from build123d import *

# Parameters (mm, degrees)
SKETCH_1_R               = 3.9
SKETCH_1_R_2             = 2.65
EXTRUDE_1_DEPTH          = 11
EXTRUDE_START            = -3
SKETCH_2_R               = 2.65
EXTRUDE_2_DEPTH          = 3
EXTRUDE_START_2          = 6.2
EXTRUDE_3_DEPTH          = 6.2
CHAMFER_1_SIZE           = 0.3
CHAMFER_2_SIZE           = 0.3
EXTRUDE_4_DEPTH          = 1
EXTRUDE_4_DEPTH_BACK     = 2
SKETCH_4_R               = 13.9
SKETCH_5_R               = 4.9
SKETCH_5_R_2             = 3.7
EXTRUDE_5_DEPTH          = 5
CHAMFER_4_SIZE           = 2
CUT_EXTRUDE_1_DEPTH      = 22.619898242
CUT_EXTRUDE_1_DEPTH_BACK = 22.619898242
SKETCH_6_R               = 1.5
CHAMFER_5_SIZE           = 1
CHAMFER_6_SIZE           = 1


with BuildPart() as part:
    # 草图1 → 凸台-拉伸1 (new body)
    with BuildSketch(Plane.XY):
        Circle(SKETCH_1_R)
        Circle(SKETCH_1_R_2, mode=Mode.SUBTRACT)
    extrude(amount=EXTRUDE_1_DEPTH)

    # 草图2 → 凸台-拉伸2 (add)
    with BuildSketch(Plane.XY.offset(11).offset(EXTRUDE_START)):
        Circle(SKETCH_2_R)
    extrude(amount=EXTRUDE_2_DEPTH)

    # 草图3 → 凸台-拉伸3 (add)
    with BuildSketch(Plane(origin=(0, 0, 8), x_dir=(-1, 0, 0), z_dir=(0, 0, -1)).offset(EXTRUDE_START_2)):
        with BuildLine():
            Line((-1.65, -2.073644135), (-1.65, 2.073644135))
            ThreePointArc((-1.65, 2.073644135), (-2.65, 0), (-1.65, -2.073644135))
        make_face()
        with BuildLine():
            ThreePointArc((2.65, 0), (2.386943652, 1.151086443), (1.65, 2.073644135))
            Line((1.65, 2.073644135), (1.65, -2.073644135))
            ThreePointArc((1.65, -2.073644135), (2.386943652, -1.151086443), (2.65, 0))
        make_face()
    extrude(amount=-EXTRUDE_3_DEPTH)

    # 倒角1
    chamfer_1_edges = [part.edges().sort_by_distance(p)[0] for p in [
        (-2.65, 0, 0),
    ]]
    chamfer(chamfer_1_edges, length=CHAMFER_1_SIZE)

    # 倒角2
    chamfer_2_edges = [part.edges().sort_by_distance(p)[0] for p in [
        (-3.9, 0, 0),
    ]]
    chamfer(chamfer_2_edges, length=CHAMFER_2_SIZE)

    # 草图4 → 凸台-拉伸4 (add, two sides: drawn at the far end of the back side and taken through both)
    with BuildSketch(Plane.XY.offset(11).offset(-EXTRUDE_4_DEPTH_BACK)):
        Circle(SKETCH_4_R)
    extrude(amount=EXTRUDE_4_DEPTH + EXTRUDE_4_DEPTH_BACK)

    # 草图5 → 凸台-拉伸5 (add)
    with BuildSketch(Plane(origin=(0, 0, 9), x_dir=(-1, 0, 0), z_dir=(0, 0, -1))):
        with Locations(Location((0, 0, 0), (0, 0, 180))):
            Circle(SKETCH_5_R)
        Circle(SKETCH_5_R_2, mode=Mode.SUBTRACT)
    extrude(amount=EXTRUDE_5_DEPTH)

    # 倒角4
    chamfer_4_edges = [part.edges().sort_by_distance(p)[0] for p in [
        (-13.9, 0, 9),
    ]]
    chamfer(chamfer_4_edges, length=CHAMFER_4_SIZE)

    # 草图6 → 切除-拉伸1 (cut, two sides: drawn at the far end of the back side and taken through both)
    with BuildSketch(Plane(origin=(0, 0, 9), x_dir=(-1, 0, 0), z_dir=(0, 0, -1)).offset(-CUT_EXTRUDE_1_DEPTH_BACK)):
        with Locations((0, 6)):
            Circle(SKETCH_6_R)
        with Locations((5.196152423, 3)):
            Circle(SKETCH_6_R)
        with Locations((5.196152423, -3)):
            Circle(SKETCH_6_R)
        with Locations((0, -6)):
            Circle(SKETCH_6_R)
        with Locations((-5.196152423, -3)):
            Circle(SKETCH_6_R)
        with Locations((-5.196152423, 3)):
            Circle(SKETCH_6_R)
    extrude(amount=CUT_EXTRUDE_1_DEPTH + CUT_EXTRUDE_1_DEPTH_BACK, mode=Mode.SUBTRACT)

    # 倒角5
    chamfer_5_edges = [part.edges().sort_by_distance(p)[0] for p in [
        (-1.65, 0, 1.8),
    ]]
    chamfer(chamfer_5_edges, length=CHAMFER_5_SIZE - 0.0001)  # a hair under: the kernel refuses the full size

    # 倒角6
    chamfer_6_edges = [part.edges().sort_by_distance(p)[0] for p in [
        (1.65, 0, 1.8),
    ]]
    chamfer(chamfer_6_edges, length=CHAMFER_6_SIZE - 0.0001)  # a hair under: the kernel refuses the full size


solid = part.part
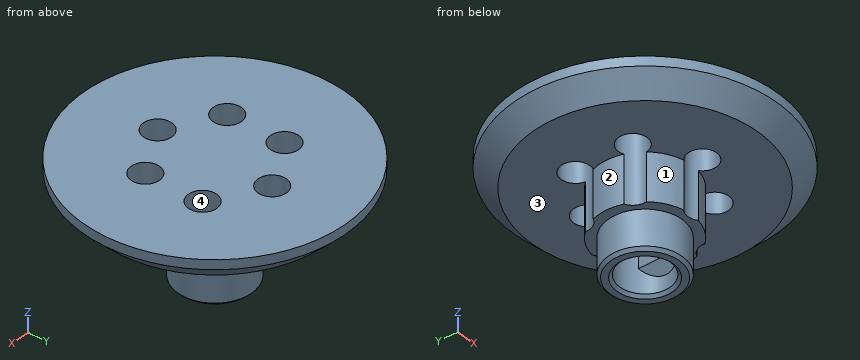
The listing builds one solid part. Answer for the finished solid, in the listing's coordinates (mm). Face numbers are marked on the shaded views. A direction names the side the tool comes from. Coordinates: 2 decimals unless noted, no trailing zeros. Order: outer loops, then holes, each group sorted by start corner. A loop starts at its lowest first (then second) coordinate and runs counter-clockwise, first axis right, second up.
Q1. Consider line 1 (Y direction, x = 0, z = 5.75); line 2 (X direction, y = 3, z = 10.25); line 3 (Y direction, x = -4.25, z = 9.75). Determine where each line is inside the solid, lowest interval first.
Q2. A cutting plane is placed at B-B, the plane z = 7. Write down the section's boundary in (x, y).
Q3. Which of the six approach directions +Z, -Z, +X, -X, +Y, -Y give full straight-line access (tool end or side, diameter ignored) to the marked faces 1, 2, 3 and 4?
Q4. A cutting plane is placed at A-A, the plane z = 9.5. Write down the section's boundary in (x, y), and give its area (3 significant figures).
Q5. Given P1, Ø4, axis at x = 5.2, y = -3, coming from the -Z side; P2, Ø1.5, axis at x = 3, z = 1.5, coming from the +Y side; P3, Ø6, axis at y = -6, z = 9, coming from the +X side; P4, Ø2.5, axis at x = 0, y = -6, coming from the +Z side, each flat-ended and moving along its own axis, determine where each tip first touches the part or whether it passes through.
Answers follow:
1. line 1: y = -4.5 to -2.65, 2.65 to 4.5
1. line 2: x = -12.8 to -6.7, -3.7 to 3.7, 6.7 to 12.8
1. line 3: y = -11.91 to -4.16, -1.84 to 1.84, 4.16 to 11.91
2. outline: (-4.63, -1.61) arc R1.5 cw to (-3.71, -3.2) arc R4.9 ccw to (-0.92, -4.81) arc R1.5 cw to (0.92, -4.81) arc R4.9 ccw to (3.71, -3.2) arc R1.5 cw to (4.63, -1.61) arc R4.9 ccw to (4.63, 1.61) arc R1.5 cw to (3.71, 3.2) arc R4.9 ccw to (0.92, 4.81) arc R1.5 cw to (-0.92, 4.81) arc R4.9 ccw to (-3.71, 3.2) arc R1.5 cw to (-4.63, 1.61) arc R4.9 ccw to start; hole (-1.65, -2.07) arc R2.65 ccw to (1.65, -2.07) - (1.65, 2.07) arc R2.65 ccw to (-1.65, 2.07) - close
3. face 1: -Z, -X, -Y
3. face 2: -Z, -X
3. face 3: -Z
3. face 4: +Z, -Z
4. outline: circle Ø24.8 at (0, 0); hole circle Ø3 at (-5.2, -3); hole circle Ø3 at (-5.2, 3); hole circle Ø3 at (0, -6); hole circle Ø3 at (0, 6); hole circle Ø3 at (5.2, -3); hole circle Ø3 at (5.2, 3)
4. area: 441 mm2
5. P1: stops at z = 4
5. P2: stops at y = 3.19
5. P3: stops at x = 13.38
5. P4: passes through
